```python
from build123d import *

# Parameters (mm, degrees)
SKETCH2_W            = 83
SKETCH2_H            = 76
BOSS_EXTRUDE1_DEPTH  = 1.66
SKETCH3_W            = 1
SKETCH3_H            = 1
CUT_EXTRUDE1_DEPTH   = 113.551124384
M3_CLEARANCE_HOLE2_D = 3.6


with BuildPart() as part:
    # Sketch2 → Boss-Extrude1 (new body)
    with BuildSketch(Plane(origin=(0, 0, 0), x_dir=(1, 0, 0), z_dir=(0, 1, 0))):
        with Locations((41.5, 38)):
            Rectangle(SKETCH2_W, SKETCH2_H)
    extrude(amount=BOSS_EXTRUDE1_DEPTH)

    # Sketch3 → Cut-Extrude1 (cut, through all)
    with BuildSketch(Plane(origin=(0, 1.66, 0), x_dir=(1, 0, 0), z_dir=(0, 1, 0))):
        with Locations((77, 38)):
            Rectangle(SKETCH3_W, SKETCH3_H)
        with Locations((77, 40.54)):
            Rectangle(SKETCH3_W, SKETCH3_H)
        with Locations((77, 35.46)):
            Rectangle(SKETCH3_W, SKETCH3_H)
    extrude(amount=-CUT_EXTRUDE1_DEPTH, mode=Mode.SUBTRACT)

    # M3 Clearance Hole2 (through all)
    with Locations(Plane(origin=(0, 1.66, 0), x_dir=(1, 0, 0), z_dir=(0, 1, 0))):
        with Locations((13, 61), (70, 61), (70, 15), (13, 15)):
            Hole(M3_CLEARANCE_HOLE2_D / 2)


solid = part.part
```
Here's how the part is built. I have some questions about the finished solid (model axes, mm). Give positions to 0.01 mm unless a question says otherwise; leave off trailing zeros. Order: outer loops, then holes, each group sorted by start corner. A loop starts at its lowest first (then second) coordinate and runs counter-clockwise, first axis right, second up. Notation, with made-up numbers: (37.5, 56.25) - (93.5, 56.25) arc R24 ccw to (93.5, 81.25) - close; hole circle Ø2 at (88.25, 77). An arc over 180 degrees is marked (long way). Answer as a JSON object with one key per item and string values. Group by question number.
Item 1: If we section it at B-B on z = -61: Please give me the cut outline in (x, y).
Item 2: If we mould it in two halves opening along X, with no side actions, what happens to faces 1 (the flat face through (41, 0, -39)), 2 (the cylindrical face through (71.327, 0.818, -16.217)), 3 (the cylindrical face through (71.327, 0.818, -62.217))? For each: pulls with the +X half, pulls with the -X half, needs draft (parallel to the pull), parting line crosses it, or undercut.
Item 3: Please list where these lines run through material, in increasing order: probe 1 along X at (y, z) = (1.2, -61); probe 2 along Z at (x, y) = (70, 1.1); probe 3 along Z at (x, y) = (11.5, 1.5).
Item 4: If we section it at A-A on x = 13: Please give me the cut outline in (y, z), and give its area (3 significant figures).
Result set:
{
 "1": {"outline": "(0, 0) - (11.2, 0) - (11.2, 1.66) - (0, 1.66) - close; (14.8, 0) - (68.2, 0) - (68.2, 1.66) - (14.8, 1.66) - close; (71.8, 0) - (83, 0) - (83, 1.66) - (71.8, 1.66) - close"},
 "2": {"face 1": "needs draft", "face 2": "undercut", "face 3": "undercut"},
 "3": {"probe 1": "0 to 11.2, 14.8 to 68.2, 71.8 to 83", "probe 2": "-76 to -62.8, -59.2 to -16.8, -13.2 to 0", "probe 3": "-76 to -61.99, -60.01 to -15.99, -14.01 to 0"},
 "4": {"outline": "(0, -76) - (1.66, -76) - (1.66, -62.8) - (0, -62.8) - close; (0, -59.2) - (1.66, -59.2) - (1.66, -16.8) - (0, -16.8) - close; (0, -13.2) - (1.66, -13.2) - (1.66, 0) - (0, 0) - close", "area": "114 mm²"}
}
